from build123d import *

# Parameters (mm, degrees)
SKETCH1_R           = 2.265
BOSS_EXTRUDE1_DEPTH = 3
SKETCH2_W           = 6.5
SKETCH2_H           = 20
CUT_EXTRUDE1_DEPTH  = 3
BOSS_EXTRUDE2_DEPTH = 3
CUT_EXTRUDE2_DEPTH  = 3
SKETCH5_W           = 3
SKETCH5_H           = 20
BOSS_EXTRUDE3_DEPTH = 3
SKETCH6_W           = 27.010134686
SKETCH6_H           = 17.9
CUT_EXTRUDE3_DEPTH  = 3
SKETCH7_W           = 19.5
SKETCH7_H           = 14.6
CUT_EXTRUDE4_DEPTH  = 3
SKETCH8_W           = 19.5
SKETCH8_H           = 15.6
CUT_EXTRUDE5_DEPTH  = 3
SKETCH9_W           = 2.019620965
SKETCH9_H           = 0.574286347
CUT_EXTRUDE6_DEPTH  = 3
FILLET1_R           = 0.6


with BuildPart() as part:
    # Sketch1 → Boss-Extrude1 (new body)
    with BuildSketch(Plane(origin=(0, 0, 0), x_dir=(1, 0, 0), z_dir=(0, 1, 0))):
        with BuildLine():
            Line((4.265, 0), (87.735, 0))
            ThreePointArc((87.735, 0), (95.015810422, 3.015810422), (92, -4.265))
            Line((92, -4.265), (92, -58.735))
            ThreePointArc((92, -58.735), (95.015810422, -66.015810422), (87.735, -63))
            Line((87.735, -63), (4.265, -63))
            ThreePointArc((4.265, -63), (-3.015810422, -66.015810422), (0, -58.735))
            Line((0, -58.735), (0, -4.265))
            ThreePointArc((0, -4.265), (-3.015810422, 3.015810422), (4.265, 0))
        make_face()
        with Locations(Location((0, 0, 0), (0, 0, 270))):
            Circle(SKETCH1_R, mode=Mode.SUBTRACT)
        with Locations(Location((92, 0, 0), (0, 0, 270))):
            Circle(SKETCH1_R, mode=Mode.SUBTRACT)
        with Locations(Location((92, -63, 0), (0, 0, 270))):
            Circle(SKETCH1_R, mode=Mode.SUBTRACT)
        with Locations(Location((0, -63, 0), (0, 0, 270))):
            Circle(SKETCH1_R, mode=Mode.SUBTRACT)
    extrude(amount=BOSS_EXTRUDE1_DEPTH)

    # Sketch2 → Cut-Extrude1 (cut)
    with BuildSketch(Plane(origin=(0, 3, 0), x_dir=(1, 0, 0), z_dir=(0, 1, 0))):
        with Locations((3.25, -31.5)):
            Rectangle(SKETCH2_W, SKETCH2_H)
    extrude(amount=-CUT_EXTRUDE1_DEPTH, mode=Mode.SUBTRACT)

    # Sketch3 → Boss-Extrude2 (add)
    with BuildSketch(Plane(origin=(0, 3, 0), x_dir=(1, 0, 0), z_dir=(0, 1, 0))):
        with BuildLine():
            Line((-2.7, -15.5), (0, -14.9))
            Line((0, -14.9), (0, -21.5))
            Line((0, -21.5), (-2.5, -21.5))
            ThreePointArc((-2.5, -21.5), (-2.853553391, -21.353553391), (-3, -21))
            Line((-3, -21), (-3, -15.8))
            ThreePointArc((-3, -15.8), (-2.912132034, -15.587867966), (-2.7, -15.5))
        make_face()
        with BuildLine():
            Line((-3, -42), (-3, -47.2))
            ThreePointArc((-3, -47.2), (-2.912132034, -47.412132034), (-2.7, -47.5))
            Line((-2.7, -47.5), (0, -48.1))
            Line((0, -48.1), (0, -41.5))
            Line((0, -41.5), (-2.5, -41.5))
            ThreePointArc((-2.5, -41.5), (-2.853553391, -41.646446609), (-3, -42))
        make_face()
    extrude(amount=-BOSS_EXTRUDE2_DEPTH)

    # Sketch4 → Cut-Extrude2 (cut)
    with BuildSketch(Plane(origin=(0, 3, 0), x_dir=(1, 0, 0), z_dir=(0, 1, 0))):
        with BuildLine():
            Line((6, -3), (64, -3))
            ThreePointArc((64, -3), (66.121320344, -3.878679656), (67, -6))
            Line((67, -6), (67, -57))
            ThreePointArc((67, -57), (66.121320344, -59.121320344), (64, -60))
            Line((64, -60), (6, -60))
            ThreePointArc((6, -60), (3.878679656, -59.121320344), (3, -57))
            Line((3, -57), (3, -6))
            ThreePointArc((3, -6), (3.878679656, -3.878679656), (6, -3))
        make_face()
    extrude(amount=-CUT_EXTRUDE2_DEPTH, mode=Mode.SUBTRACT)

    # Sketch5 → Boss-Extrude3 (add)
    with BuildSketch(Plane(origin=(0, 3, 0), x_dir=(1, 0, 0), z_dir=(0, 1, 0))):
        with Locations((1.5, -31.5)):
            Rectangle(SKETCH5_W, SKETCH5_H)
    extrude(amount=-BOSS_EXTRUDE3_DEPTH)

    # Sketch6 → Cut-Extrude3 (cut)
    with BuildSketch(Plane(origin=(0, 3, 0), x_dir=(1, 0, 0), z_dir=(0, 1, 0))):
        with Locations((82.505067343, -14.45)):
            Rectangle(SKETCH6_W, SKETCH6_H)
    extrude(amount=-CUT_EXTRUDE3_DEPTH, mode=Mode.SUBTRACT)

    # Sketch7 → Cut-Extrude4 (cut)
    with BuildSketch(Plane(origin=(0, 3, 0), x_dir=(1, 0, 0), z_dir=(0, 1, 0))):
        with Locations((82.25, -33.7)):
            Rectangle(SKETCH7_W, SKETCH7_H)
    extrude(amount=-CUT_EXTRUDE4_DEPTH, mode=Mode.SUBTRACT)

    # Sketch8 → Cut-Extrude5 (cut)
    with BuildSketch(Plane(origin=(0, 3, 0), x_dir=(1, 0, 0), z_dir=(0, 1, 0))):
        with Locations((82.25, -51.3)):
            Rectangle(SKETCH8_W, SKETCH8_H)
    extrude(amount=-CUT_EXTRUDE5_DEPTH, mode=Mode.SUBTRACT)

    # Sketch9 → Cut-Extrude6 (cut)
    with BuildSketch(Plane(origin=(0, 3, 0), x_dir=(1, 0, 0), z_dir=(0, 1, 0))):
        with Locations((93.009810483, -58.812856827)):
            Rectangle(SKETCH9_W, SKETCH9_H)
    extrude(amount=-CUT_EXTRUDE6_DEPTH, mode=Mode.SUBTRACT)

    # Fillet1
    fillet1_edges = [part.edges().sort_by_distance(p)[0] for p in [
        (0, 1.5, 41.5),
        (92, 1.5, 4.265),
        (0, 1.5, 21.5),
        (87.735, 1.5, 63),
        (4.265, 1.5, 63),
        (0, 1.5, 58.735),
        (0, 1.5, 4.265),
        (4.265, 1.5, 0),
        (87.735, 1.5, 0),
        (93.726332818, 1.5, 59.1),
        (0, 1.5, 14.9),
        (0, 1.5, 48.1),
    ]]
    fillet(fillet1_edges, radius=FILLET1_R)


solid = part.part
CAD build for the part. Positions are in the model's coordinates, mm. A direction names the side the tool comes from. Give positions to 0.01 mm unless a question says otherwise; leave off trailing zeros. Order: outer loops, then holes, each group sorted by start corner. A loop starts at its lowest first (then second) coordinate and runs counter-clockwise, first axis right, second up. Notation, with made-up numbers: (-22.5, 57.25) - (24.5, 57.25) arc R12 cw to (24.5, 76.25) - close; hole circle Ø10 at (-27.75, -30). An arc over 180 degrees is marked (long way). Answer in a Markdown table with one row per item.
1. Saw through at C-C, the plane y = 1. Count the separate pieces of the cut face and the enclosed holes in it, plus the area to 3 significant figures.
Data:
| item | result |
|---|---|
| separate pieces | 1 |
| enclosed holes | 5 |
| area | 1,300 mm² |
2. Probe probe 1 along Z at (x, y) = (87, 0.65); probe 2 along Z at (x, y) = (51, 1.5); probe 3 along Z at (x, y) = (70, 0.7). List the from-to ranges inside material, lowest first. Write a range as [from, to].
Data:
| item | result |
|---|---|
| probe 1 | z = [0, 5.5], [23.4, 26.4], [41, 43.5], [59.1, 63] |
| probe 2 | z = [0, 3], [60, 63] |
| probe 3 | z = [0, 5.5], [23.4, 63] |
3. Saw through at B-B, the plane x = 85.5. Give the cut face in (y, z).
Data:
| item | result |
|---|---|
| outline | (0, 0) - (3, 0) - (3, 5.5) - (0, 5.5) - close; (0, 23.4) - (3, 23.4) - (3, 26.4) - (0, 26.4) - close; (0, 41) - (3, 41) - (3, 43.5) - (0, 43.5) - close; (0, 59.1) - (3, 59.1) - (3, 63) - (0, 63) - close |
4. Saw through at A-A, the plane x = 56.5. Give the cut face in (y, z).
Data:
| item | result |
|---|---|
| outline | (0, 0) - (3, 0) - (3, 3) - (0, 3) - close; (0, 60) - (3, 60) - (3, 63) - (0, 63) - close |
5. Pull direction X, two halves, no side cores. Call faces 1 (the flat face through (0, 2, 32)), 2 (the cylindrical face through (-3.11, 1.48, -2.92)), 3 (the flat face through (82, 2, 41)): pulls with the +X half, pulls with the -X half, needs draft (parallel to the pull), parting line crosses it, or undercut.
Data:
| item | result |
|---|---|
| face 1 | pulls with the -X half |
| face 2 | undercut |
| face 3 | needs draft |
6. Flat gauge pins, fed straight in: pin 1 (0.9 mm diameter, centred on x = 86, y = 1.5, fed in from +Z); pin 2 (0.9 mm diameter, centred on y = 2, z = 19, fed in from +X); pin 3 (0.9 mm diameter, centred on y = 2, z = 28, fed in from -X). Where does each tip first touch, or does it go through?
Data:
| item | result |
|---|---|
| pin 1 | stops at z = 63 |
| pin 2 | stops at x = 69 |
| pin 3 | stops at x = 0 |
7. Tool access for faces 4 (the flat face through (69, 2, 15)), 5 (the flat face through (0, 1, 53)), 6 (the flat face through (47, 1, 63)), 7 (the flat face through (35, 2, 3)): list every direction of +Z, -Z, +X, -X, +Y, -Y with a clear straight run to the whole face (end or side of a thin tool).
Data:
| item | result |
|---|---|
| face 4 | +X, +Y, -Y |
| face 5 | -X, +Y, -Y |
| face 6 | +Z, +Y, -Y |
| face 7 | +Y, -Y |
